Verification items for the finished model (mm, model axes). Give positions to 0.01 mm unless a question says otherwise; leave off trailing zeros. Write each loop counter-clockwise with the first axis right and the second up, starting at its lowest first coordinate (ties: lowest second). Pieces come first, ordered by that corner, then holes. Notation, with made-up numbers: (57.25, 66) -> (85.25, 66) arc R27 cw to (85.25, 85) -> close; hole circle Ø5 at (31.5, -32). An arc over 180 degrees is marked (long way). Use CSV: the item, a comma, the result in double quotes. Start each with the question number.
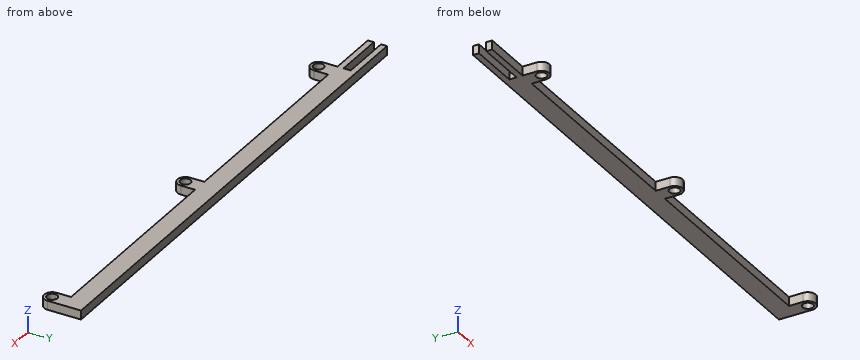
```python
from build123d import *

# Parameters (mm, degrees)
F0_W     = 259.72
F0_H     = 6.4
F1_DEPTH = 3
F3_DEPTH = 3
F4_R     = 2.63999
F5_W     = 17.32
F5_H     = 2.4
F6_DEPTH = 3.001


# Not quite as in the source:
# - a fillet or chamfer is up to 0.001 mm smaller than in the source, because OpenCascade refuses the exact size


with BuildPart() as f1:
    # F0 (on Top) → F1 (new body)
    with BuildSketch(Plane.XY):
        Rectangle(F0_W, F0_H)
    extrude(amount=F1_DEPTH)

    # F2 (on Top) → F3 (join)
    with BuildSketch(Plane.XY):
        with BuildLine():
            Line((129.86, -10.59), (129.86, -3.2))
            Line((129.86, -3.2), (124.58, -3.2))
            Line((124.58, -3.2), (124.58, -7.95))
            Line((124.58, -7.95), (125.47, -7.95))
            ThreePointArc((125.47, -7.95), (127.22, -6.2), (128.97, -7.95))
            ThreePointArc((128.97, -7.95), (128.4574368671, -9.1874368671), (127.22, -9.7))
            Line((127.22, -9.7), (127.22, -10.59))
            Line((127.22, -10.59), (129.86, -10.59))
        make_face()
        with BuildLine():
            Line((125.47, -7.95), (124.58, -7.95))
            Line((124.58, -7.95), (124.58, -10.59))
            Line((124.58, -10.59), (127.22, -10.59))
            Line((127.22, -10.59), (127.22, -9.7))
            ThreePointArc((127.22, -9.7), (125.9825631329, -9.1874368671), (125.47, -7.95))
        make_face()
        Polygon((53.66, -10.59), (53.66, -3.2), (48.38, -3.2), (48.38, -7.95), (48.38, -10.59), align=None)
        with BuildLine():
            ThreePointArc((52.77, -7.95), (51.02, -9.7), (49.27, -7.95))
            ThreePointArc((49.27, -7.95), (51.02, -6.2), (52.77, -7.95))
        make_face(mode=Mode.SUBTRACT)
        Polygon((-22.54, -3.2), (-27.82, -3.2), (-27.82, -7.95), (-27.82, -10.59), (-22.54, -10.59), align=None)
        with BuildLine():
            ThreePointArc((-23.43, -7.95), (-25.18, -9.7), (-26.93, -7.95))
            ThreePointArc((-26.93, -7.95), (-25.18, -6.2), (-23.43, -7.95))
        make_face(mode=Mode.SUBTRACT)
    extrude(amount=F3_DEPTH)

    # F4 (radius 2.64 in the source; OpenCascade refuses exactly that, so slightly less here)
    f4_edges = [f1.edges().sort_by_distance(p)[0] for p in [
        (48.38, -10.59, 1.5),
        (53.66, -10.59, 1.5),
        (124.58, -10.59, 1.5),
        (129.86, -10.59, 1.5),
        (-27.82, -10.59, 1.5),
        (-22.54, -10.59, 1.5),
    ]]
    fillet(f4_edges, radius=F4_R)

    # F5 (on face) → F6 (cut, through all)
    with BuildSketch(Plane.XY.offset(3)):
        Polygon((-45.14, 3.2), (-129.86, 3.2), (-129.86, -3.2), (-45.14, -3.2), (-45.14, -1.2), (-45.14, 1.2), align=None)
        with Locations((-36.48, 0)):
            Rectangle(F5_W, F5_H)
    extrude(amount=-F6_DEPTH, mode=Mode.SUBTRACT)


solid = f1.part
```
(1) Section check B-B on x = 108. Record the cut outline in (y, z), then the cut area to 3 significant figures.
(2) Thickness scan on line 1 (X direction, y = -5.75, z = 0.4); line 2 (X direction, y = -8.5, z = 2.95); line 3 (Y direction, x = 17, z = 2.3). Record the ranges inside material, lowest first. Write a range as from..to.
(3) Section check A-A on z = 2.55. Give the number of separate pieces and of enclosed holes in the cut face, then the cut area to 3 significant figures.
(4) Go/stop test with flat-tipped pins: pin 1 (1.5 mm diameter, centred on x = 85, z = 1, fed in from -Y); pin 2 (2 mm diameter, centred on x = -7, y = -5.5, fed in from +Z); pin 3 (1.5 mm diameter, centred on y = -8, z = 1, fed in from -X); pin 4 (8 mm diameter, centred on x = 86.5, y = -1.5, fed in from -Z). Record where each tip stops, or that it passes through.
Data:
1,outline,"(-3.2, 0) -> (3.2, 0) -> (3.2, 3) -> (-3.2, 3) -> close"
1,area,"19.2 mm2"
2,line 1,"x = -27.82..-22.54, 48.38..53.66, 124.58..129.86"
2,line 2,"x = -27.76..-26.84, -23.52..-22.6, 48.44..49.36, 52.68..53.6, 124.64..125.56, 128.88..129.8"
2,line 3,"y = -3.2..3.2"
3,separate pieces,"1"
3,enclosed holes,"3"
3,area,"1,160 mm2"
4,pin 1,"stops at y = -3.2"
4,pin 2,"passes through"
4,pin 3,"stops at x = -27.82"
4,pin 4,"stops at z = 0"
